Geometry: final body of the model. Coordinates: model frame, mm. Face numbers are marked on the shaded views. A direction names the side the tool comes from. Give positions to 0.01 mm unless a question says otherwise; leave off trailing zeros. Write each loop counter-clockwise with the first axis right and the second up, starting at its lowest first coordinate (ties: lowest second). Pieces come first, ordered by that corner, then holes. Notation, with made-up numbers: M -7,-40 L 6,-40 A21 ccw 6,-15 Z; hole C -0.75,28 d5. An arc over 180 degrees is marked long. Use a Markdown table: item, result. Add a question column.
1) Line query: line 1 (Z direction, x = 4.5, y = -1); line 2 (X direction, y = -0.25, z = -67); line 3 (X direction, y = -2.75, z = -57). Output: solid intervals per line, ascending.
2) Section A-A on x = 0. Return the cut outline in (y, z), then the cut area to 3 significant figures.
3) Section B-B on z = -15. Return the cut outline in (x, y), then the cut area to 3 significant figures.
4) Set-up query: the marked faces 1 and 2. Return all of +Z, -Z, +X, -X, +Y, -Y with unobstructed straight access to the full face (end or side cutting, diameter ignored); none if empty.
5) Pin query (flat end, axial travel): pin 1 (4 mm diameter, centred on y = -3, z = -51.5, fed in from +X); pin 2 (6 mm diameter, centred on y = 0.5, z = -37.5, fed in from -X); pin 3 (1 mm diameter, centred on x = -2, z = -45, fed in from +Y). Return the tip coordinate at first contact, or that it passes through.
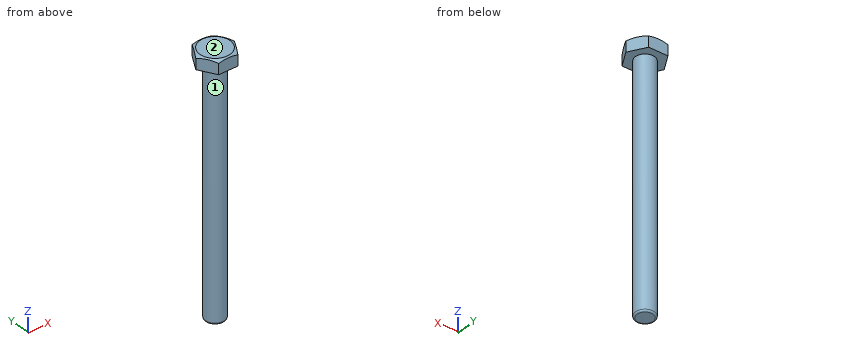
```python
from build123d import *

# Parameters (mm, degrees)
BOSS_EXTRUDE1_DEPTH = 4
SKETCH5_R           = 3
BOSS_EXTRUDE2_DEPTH = 76
FILLET1_R           = 0.5


with BuildPart() as part:
    # Sketch1 → Boss-Extrude1 (new body)
    with BuildSketch(Plane.XY):
        Polygon((6, 0), (3, 5.196152423), (-3, 5.196152423), (-6, 0), (-3, -5.196152423), (3, -5.196152423), align=None)
    extrude(amount=BOSS_EXTRUDE1_DEPTH)

    # Sketch4 → Cut-Revolve1 (revolve, cut)
    with BuildSketch(Plane(origin=(0, 0, 0), x_dir=(0, 0, -1), z_dir=(0.866025404, 0.5, 0))):
        Polygon((-4, 4.729715048), (-3.3, 6), (-4, 6), align=None)
    revolve(axis=Axis((0, 0, 6.225223698), (0, 0, -1)), mode=Mode.SUBTRACT)

    # Sketch5 → Boss-Extrude2 (add)
    with BuildSketch(Plane(origin=(0, 0, 0), x_dir=(-1, 0, 0), z_dir=(0, 0, -1))):
        Circle(SKETCH5_R)
    extrude(amount=BOSS_EXTRUDE2_DEPTH)

    # Fillet1
    fillet1_edges = [part.edges().sort_by_distance(p)[0] for p in [
        (3, 0, -76),
    ]]
    fillet(fillet1_edges, radius=FILLET1_R)


solid = part.part
```
Found:
| question | item | result |
|---|---|---|
| 1 | line 1 | 0 to 4 |
| 1 | line 2 | -2.99 to 2.99 |
| 1 | line 3 | -1.2 to 1.2 |
| 2 | outline | M -5.2,0 L -3,0 L -3,-75.5 A0.5 ccw -2.5,-76 L 2.5,-76 A0.5 ccw 3,-75.5 L 3,0 L 5.2,0 L 5.2,3.74 L 4.73,4 L -4.73,4 L -5.2,3.74 Z |
| 2 | area | 497 mm² |
| 3 | outline | C 0,0 d6 |
| 3 | area | 28.3 mm² |
| 4 | face 1 | -Z |
| 4 | face 2 | +Z, +X, -X, +Y, -Y |
| 5 | pin 1 | x = 2.83 |
| 5 | pin 2 | x = -3 |
| 5 | pin 3 | y = 2.6 |
